```python
from build123d import *
from build123d.topology import SkipClean

# Parameters (mm, degrees)
SKETCH1_W             = 48
SKETCH1_H             = 53
BOSS_EXTRUDE1_DEPTH   = 10
SKETCH2_W             = 48
SKETCH2_H             = 5.616325
BOSS_EXTRUDE2_DEPTH   = 33.1917878
SKETCH4_W             = 4
SKETCH4_H             = 10
BOSS_EXTRUDE4_DEPTH   = 40
SKETCH5_W             = 48
SKETCH5_H             = 10.8609375
BOSS_EXTRUDE5_DEPTH   = 23.1917878
SKETCH6_W             = 48
SKETCH6_H             = 5
BOSS_EXTRUDE6_DEPTH   = 42.3
SKETCH7_W             = 12.8082122
SKETCH7_H             = 16.4772625
BOSS_EXTRUDE7_DEPTH   = 48
CUT_EXTRUDE1_REACH    = 84.426
SKETCH8_R             = 11.5
SKETCH8_R_2           = 2
FILLET1_R             = 10
FILLET2_R             = 4
SKETCH9_W             = 5
SKETCH9_H             = 16.4772625
BOSS_EXTRUDE9_DEPTH   = 48
CUT_EXTRUDE2_DEPTH    = 88.252507127
SKETCH11_W            = 51
SKETCH11_H            = 16.4772625
BOSS_EXTRUDE10_DEPTH  = 49.45
BOSS_EXTRUDE11_DEPTH  = 46
SKETCH16_W            = 47.95
SKETCH16_H            = 51
BOSS_EXTRUDE14_DEPTH  = 2.55
SKETCH14_W            = 5
SKETCH14_H            = 42.3
BOSS_EXTRUDE13_DEPTH  = 1.5
SKETCH17_W            = 51
SKETCH17_H            = 19.0272625
BOSS_EXTRUDE15_DEPTH  = 9
BOSS_EXTRUDE16_DEPTH  = 25
SKETCH19_R            = 1.9304
CUT_EXTRUDE3_DEPTH    = 125.404890183
MIRROR2_START         = 33.1917878
MIRROR2_DEPTH         = 51
MIRROR2_START_2       = 76.1917878
MIRROR2_2_OUTLINE_W   = 47.95
MIRROR2_2_OUTLINE_H   = 25
MIRROR2_2_OUTLINE_R   = 1.9304
MIRROR2_2_DEPTH       = 8
MIRROR2_3_OUTLINE_W   = 45
MIRROR2_3_OUTLINE_H   = 42.3
MIRROR2_3_OUTLINE_R   = 2
MIRROR2_3_OUTLINE_R_2 = 11.5
MIRROR2_3_DEPTH       = 5
SKETCH20_W            = 103.287975037
SKETCH20_H            = 97.84889924
CUT_EXTRUDE4_DEPTH    = 144.929961559
SKETCH21_W            = 49.5
SKETCH21_H            = 42.3
CUT_EXTRUDE5_DEPTH    = 128.391431036
SKETCH24_R            = 7.5
BOSS_EXTRUDE18_DEPTH  = 45
BOSS_EXTRUDE19_DEPTH  = 29


# Read off the part's stored shape, not the designer's step: Mirror2
with BuildPart() as part:
    # Sketch1 → Boss-Extrude1 (new body)
    with BuildSketch(Plane.XY):
        with Locations((24, 26.5)):
            Rectangle(SKETCH1_W, SKETCH1_H)
    extrude(amount=BOSS_EXTRUDE1_DEPTH)

    # Sketch2 → Boss-Extrude2 (add)
    with BuildSketch(Plane(origin=(0, 0, 0), x_dir=(-1, 0, 0), z_dir=(0, 0, -1))):
        with Locations((-24, -2.8081625)):
            Rectangle(SKETCH2_W, SKETCH2_H)
    extrude(amount=-BOSS_EXTRUDE2_DEPTH)

    # Sketch4 → Boss-Extrude4 (add)
    with BuildSketch(Plane.XY.offset(10)):
        with Locations((2, 48)):
            Rectangle(SKETCH4_W, SKETCH4_H)
        with Locations((46, 48)):
            Rectangle(SKETCH4_W, SKETCH4_H)
    extrude(amount=BOSS_EXTRUDE4_DEPTH)

    # Sketch5 → Boss-Extrude5 (add)
    with BuildSketch(Plane.XY.offset(10)):
        with Locations((24, 5.43046875)):
            Rectangle(SKETCH5_W, SKETCH5_H)
    extrude(amount=BOSS_EXTRUDE5_DEPTH)

    # Sketch6 → Boss-Extrude6 (add)
    with BuildSketch(Plane.XZ.offset(5.616325)):
        with Locations((24, 30.6917878)):
            Rectangle(SKETCH6_W, SKETCH6_H)
    extrude(amount=BOSS_EXTRUDE6_DEPTH)

    # Sketch7 → Boss-Extrude7 (add)
    with BuildSketch(Plane.ZY):
        with Locations((-6.4041061, 2.62230625)):
            Rectangle(SKETCH7_W, SKETCH7_H)
    extrude(amount=-BOSS_EXTRUDE7_DEPTH)

    # Sketch8 → Cut-Extrude1 (cut, up to next)
    with BuildSketch(Plane(origin=(0, 0, 28.1917878), x_dir=(-1, 0, 0), z_dir=(0, 0, -1)), mode=Mode.PRIVATE) as cut_extrude1_sk1:
        with Locations((-24, -26.616325)):
            Circle(SKETCH8_R)
    cut_extrude1_tool1 = extrude(cut_extrude1_sk1.sketch, amount=-CUT_EXTRUDE1_REACH, mode=Mode.PRIVATE) & part.part
    # Sketch8 → Cut-Extrude1 (cut, up to next)
    with BuildSketch(Plane(origin=(0, 0, 28.1917878), x_dir=(-1, 0, 0), z_dir=(0, 0, -1)), mode=Mode.PRIVATE) as cut_extrude1_sk2:
        with Locations((-39.5, -11.116325)):
            Circle(SKETCH8_R_2)
    cut_extrude1_tool2 = extrude(cut_extrude1_sk2.sketch, amount=-CUT_EXTRUDE1_REACH, mode=Mode.PRIVATE) & part.part
    # Sketch8 → Cut-Extrude1 (cut, up to next)
    with BuildSketch(Plane(origin=(0, 0, 28.1917878), x_dir=(-1, 0, 0), z_dir=(0, 0, -1)), mode=Mode.PRIVATE) as cut_extrude1_sk3:
        with Locations((-39.5, -42.116325)):
            Circle(SKETCH8_R_2)
    cut_extrude1_tool3 = extrude(cut_extrude1_sk3.sketch, amount=-CUT_EXTRUDE1_REACH, mode=Mode.PRIVATE) & part.part
    # Sketch8 → Cut-Extrude1 (cut, up to next)
    with BuildSketch(Plane(origin=(0, 0, 28.1917878), x_dir=(-1, 0, 0), z_dir=(0, 0, -1)), mode=Mode.PRIVATE) as cut_extrude1_sk4:
        with Locations((-8.5, -11.116325)):
            Circle(SKETCH8_R_2)
    cut_extrude1_tool4 = extrude(cut_extrude1_sk4.sketch, amount=-CUT_EXTRUDE1_REACH, mode=Mode.PRIVATE) & part.part
    # Sketch8 → Cut-Extrude1 (cut, up to next)
    with BuildSketch(Plane(origin=(0, 0, 28.1917878), x_dir=(-1, 0, 0), z_dir=(0, 0, -1)), mode=Mode.PRIVATE) as cut_extrude1_sk5:
        with Locations((-8.5, -42.116325)):
            Circle(SKETCH8_R_2)
    cut_extrude1_tool5 = extrude(cut_extrude1_sk5.sketch, amount=-CUT_EXTRUDE1_REACH, mode=Mode.PRIVATE) & part.part
    add(cut_extrude1_tool1.solids().sort_by_distance((24, -26.616325, 28.191788))[0], mode=Mode.SUBTRACT)
    add(cut_extrude1_tool2.solids().sort_by_distance((39.5, -11.116325, 28.191788))[0], mode=Mode.SUBTRACT)
    add(cut_extrude1_tool3.solids().sort_by_distance((39.5, -42.116325, 28.191788))[0], mode=Mode.SUBTRACT)
    add(cut_extrude1_tool4.solids().sort_by_distance((8.5, -11.116325, 28.191788))[0], mode=Mode.SUBTRACT)
    add(cut_extrude1_tool5.solids().sort_by_distance((8.5, -42.116325, 28.191788))[0], mode=Mode.SUBTRACT)

    # Fillet1
    fillet1_edges = [part.edges().sort_by_distance(p)[0] for p in [
        (24, 10.8609375, 0),
    ]]
    fillet(fillet1_edges, radius=FILLET1_R)

    # Fillet2
    fillet2_edges = [part.edges().sort_by_distance(p)[0] for p in [
        (2, 43, 10),
        (46, 43, 10),
    ]]
    fillet(fillet2_edges, radius=FILLET2_R)

    # Sketch9 → Boss-Extrude9 (add)
    with BuildSketch(Plane(origin=(48, 0, 0), x_dir=(0, 0, -1), z_dir=(1, 0, 0))):
        with Locations((15.3082122, 2.62230625)):
            Rectangle(SKETCH9_W, SKETCH9_H)
    extrude(amount=-BOSS_EXTRUDE9_DEPTH)

    # Sketch10 → Cut-Extrude2 (cut, through all)
    with BuildSketch(Plane(origin=(48, 0, 0), x_dir=(0, 0, -1), z_dir=(1, 0, 0))):
        Polygon((17.8082122, 10.8609375), (-33.1917878, 10.8609375), (-76.887145623, 43.902095521), (-50.794096938, 74.436514195), (27.207463492, 71.105486703), align=None)
    extrude(amount=-CUT_EXTRUDE2_DEPTH, mode=Mode.SUBTRACT)

    # Sketch11 → Boss-Extrude10 (add)
    with BuildSketch(Plane(origin=(48, 0, 0), x_dir=(0, 0, -1), z_dir=(1, 0, 0))):
        with Locations((-7.6917878, 2.62230625)):
            Rectangle(SKETCH11_W, SKETCH11_H)
    extrude(amount=BOSS_EXTRUDE10_DEPTH)

    # Sketch12 → Boss-Extrude11 (add)
    with BuildSketch(Plane(origin=(0, 0, 28.1917878), x_dir=(-1, 0, 0), z_dir=(0, 0, -1))):
        Polygon((-48, -47.916325), (-45, -47.916325), (-45, -5.616325), (-49.5, -5.616325), (-49.5, -47.916325), align=None)
    extrude(amount=BOSS_EXTRUDE11_DEPTH)

    # Sketch16 → Boss-Extrude14 (add)
    with BuildSketch(Plane.XZ.offset(5.616325)):
        with Locations((73.475, 7.6917878)):
            Rectangle(SKETCH16_W, SKETCH16_H)
    extrude(amount=BOSS_EXTRUDE14_DEPTH)

    # Sketch14 → Boss-Extrude13 (add)
    with BuildSketch(Plane(origin=(49.5, 0, 0), x_dir=(0, 0, -1), z_dir=(1, 0, 0))):
        with Locations((-30.6917878, -26.766325)):
            Rectangle(SKETCH14_W, SKETCH14_H)
    extrude(amount=-BOSS_EXTRUDE13_DEPTH)

    # Sketch17 → Boss-Extrude15 (add)
    with BuildSketch(Plane(origin=(97.45, 0, 0), x_dir=(0, 0, -1), z_dir=(1, 0, 0))):
        with Locations((-7.6917878, 1.34730625)):
            Rectangle(SKETCH17_W, SKETCH17_H)
    extrude(amount=BOSS_EXTRUDE15_DEPTH)

    # Sketch18 → Boss-Extrude16 (add)
    with BuildSketch(Plane.XZ.offset(8.166325)):
        Polygon((49.5, -17.8082122), (106.45, -17.8082122), (106.45, -9.8082122), (106.45, 33.1917878), (97.45, 33.1917878), (97.45, -9.8082122), (49.5, -9.8082122), align=None)
    extrude(amount=BOSS_EXTRUDE16_DEPTH)

    # Sketch19 → Cut-Extrude3 (cut, through all)
    with BuildSketch(Plane.XY.offset(-9.8082122)):
        with Locations((58.475, -26.166325)):
            Circle(SKETCH19_R)
        with Locations((88.475, -26.166325)):
            Circle(SKETCH19_R)
    extrude(amount=-CUT_EXTRUDE3_DEPTH, mode=Mode.SUBTRACT)

    # Mirror2 outline → Mirror2 (add)
    with BuildSketch(Plane.XY.offset(MIRROR2_START)):
        Polygon((49.5, -47.916325), (49.5, -8.166325), (97.45, -8.166325), (97.45, -33.166325), (106.45, -33.166325), (106.45, 10.8609375), (0, 10.8609375), (0, -5.616325), (45, -5.616325), (45, -47.916325), align=None)
    extrude(amount=MIRROR2_DEPTH)

    # Mirror2 2 outline → Mirror2 2 (add)
    with BuildSketch(Plane.XY.offset(MIRROR2_START_2)):
        with Locations((73.475, -20.666325)):
            Rectangle(MIRROR2_2_OUTLINE_W, MIRROR2_2_OUTLINE_H)
        with Locations((58.475, -26.166325)):
            Circle(MIRROR2_2_OUTLINE_R, mode=Mode.SUBTRACT)
        with Locations((88.475, -26.166325)):
            Circle(MIRROR2_2_OUTLINE_R, mode=Mode.SUBTRACT)
    extrude(amount=MIRROR2_2_DEPTH)

    # Mirror2 3 outline → Mirror2 3 (add)
    with SkipClean():  # the faces are left unmerged after this step: merging them gives an invalid solid
        with BuildSketch(Plane.XY.offset(MIRROR2_START)):
            with Locations((22.5, -26.766325)):
                Rectangle(MIRROR2_3_OUTLINE_W, MIRROR2_3_OUTLINE_H)
            with Locations((8.5, -42.116325)):
                Circle(MIRROR2_3_OUTLINE_R, mode=Mode.SUBTRACT)
            with Locations((39.5, -42.116325)):
                Circle(MIRROR2_3_OUTLINE_R, mode=Mode.SUBTRACT)
            with Locations((24, -26.616325)):
                Circle(MIRROR2_3_OUTLINE_R_2, mode=Mode.SUBTRACT)
            with Locations((8.5, -11.116325)):
                Circle(MIRROR2_3_OUTLINE_R, mode=Mode.SUBTRACT)
            with Locations((39.5, -11.116325)):
                Circle(MIRROR2_3_OUTLINE_R, mode=Mode.SUBTRACT)
        extrude(amount=MIRROR2_3_DEPTH)

    # Sketch20 → Cut-Extrude4 (cut, through all)
    with BuildSketch(Plane.ZY):
        with Locations((-18.452199719, -38.06351212)):
            Rectangle(SKETCH20_W, SKETCH20_H)
    extrude(amount=-CUT_EXTRUDE4_DEPTH, mode=Mode.SUBTRACT)

    # Sketch21 → Cut-Extrude5 (cut, through all)
    with BuildSketch(Plane.XY.offset(84.1917878)):
        with Locations((24.75, -26.766325)):
            Rectangle(SKETCH21_W, SKETCH21_H)
    extrude(amount=-CUT_EXTRUDE5_DEPTH, mode=Mode.SUBTRACT)



with BuildPart() as body_2:
    # Sketch24 → Boss-Extrude18 (new body)
    with BuildSketch(Plane.XY.offset(55.1917878)):
        with Locations((24, -29.616325)):
            Circle(SKETCH24_R)
    extrude(amount=-BOSS_EXTRUDE18_DEPTH)


with BuildPart() as part_1:
    add(part.part)

    add(body_2.part)  # Boss-Extrude19 merges body 2
    # Sketch25 → Boss-Extrude19 (add)
    with BuildSketch(Plane.XY.offset(55.1917878)):
        with BuildLine():
            Line((16.5, -29.616325), (12.268152463, -5.616325))
            Line((12.268152463, -5.616325), (35.731847537, -5.616325))
            Line((35.731847537, -5.616325), (31.5, -29.616325))
            ThreePointArc((31.5, -29.616325), (24, -37.116325), (16.5, -29.616325))
        make_face()
    extrude(amount=BOSS_EXTRUDE19_DEPTH)


solid = part_1.part
```
Work out the finished part from the listing and answer in its coordinate system (mm). A direction names the side the tool comes from. Coordinates: 2 decimals unless noted, no trailing zeros. Loops run counter-clockwise (first coordinate to the right, second up) from the corner with the lowest first, then second, coordinate; pieces in that order, holes last. Notation, with made-up numbers: (79, 11) -> (127, 11) arc R25 cw to (127, 32) -> close; hole circle Ø5 at (22.5, 36.5). An arc over 180 degrees is marked (long way). Answer as CSV lines item,"result".
Q1. The part is cut by section C-C on x = 71.5. Write down the section's boundary in (y, z), and give its area (3 significant figures).
Findings:
outline,"(-33.17, 76.19) -> (-8.17, 76.19) -> (-8.17, 33.19) -> (10.86, 33.19) -> (10.86, 84.19) -> (-33.17, 84.19) -> close"
area,"1,170 mm²"
Q2. The part is cut by section A-A on z = 43.5. Write down the section's boundary in (x, y).
Findings:
outline,"(0, -5.62) -> (49.5, -5.62) -> (49.5, -8.17) -> (97.45, -8.17) -> (97.45, -33.17) -> (106.45, -33.17) -> (106.45, 10.86) -> (0, 10.86) -> close; circle Ø15 at (24, -29.62)"
Q3. Find the intervals of material crossed by probe 1 along X at (y, z) = (-16, 41); probe 2 along Z at (x, y) = (101, -22); probe 3 along Y at (x, z) = (63, 40), in increasing order.
Findings:
probe 1,"x = 97.45 to 106.45"
probe 2,"z = 33.19 to 84.19"
probe 3,"y = -8.17 to 10.86"
Q4. For a pull along Y with two mould halves and no side action, classify faces 1 (the face through (86, -33.166, 77)), 2 (the face through (54, 10.861, 58)), 3 (the face through (97.45, -20, 54)), 4 (the face through (23.024, -37.053, 38.452)) as +Y half, -Y half, draft (parallel to the pull), parting line (faces both ways), or undercut.
Findings:
face 1,"-Y half"
face 2,"+Y half"
face 3,"draft"
face 4,"undercut"
Q5. The part is cut by section B-B on y = -17. Write down the section's boundary in (x, z).
Findings:
outline,"(14.28, 55.19) -> (33.72, 55.19) -> (33.72, 84.19) -> (14.28, 84.19) -> close; (49.5, 76.19) -> (97.45, 76.19) -> (97.45, 33.19) -> (106.45, 33.19) -> (106.45, 84.19) -> (49.5, 84.19) -> close"
Q6. Each of these flat-tipped pins is pushed along its axis until it touches: pin 1 (14 mm diameter, centred on y = -22, z = 62, fed in from -X); pin 2 (7.5 mm diameter, centred on x = 74, y = -26.5, fed in from -Z); pin 3 (6 mm diameter, centred on x = 82, y = 0, fed in from -Z); pin 4 (3.5 mm diameter, centred on x = 58.48, y = -26.17, fed in from +Z). Where does it stop, or does it pass through?
Findings:
pin 1,"stops at x = 13.92"
pin 2,"stops at z = 76.19"
pin 3,"stops at z = 33.19"
pin 4,"passes through"
Q7. The part is cut by section D-D on z = 61.5. Write down the section's boundary in (x, y).
Findings:
outline,"(0, -5.62) -> (12.27, -5.62) -> (16.5, -29.62) arc R7.5 ccw to (31.5, -29.62) -> (35.73, -5.62) -> (49.5, -5.62) -> (49.5, -8.17) -> (97.45, -8.17) -> (97.45, -33.17) -> (106.45, -33.17) -> (106.45, 10.86) -> (0, 10.86) -> close"
Q8. A tool of negligible diameter and unlimited length cuts with its end or side. For faces 5 (the face through (0, 3, 58)), 6 (the face through (24, -5.616, 53)), 7 (the face through (73, -8.166, 54)), 8 (the face through (49.5, -15, 78)), from which of +Z, -Z, +X, -X, +Y, -Y can it reach the whole face along a straight path? Write none if from no direction.
Findings:
face 5,"+Z, -Z, -X, +Y, -Y"
face 6,"-Z"
face 7,"-Z, -Y"
face 8,"+Z, -Z, -Y"
